```python
from build123d import *

# Parameters (mm, degrees)
SKETCH5_W             = 29.1
SKETCH5_H             = 16.3
SKETCH5_W_2           = 23.1
SKETCH5_H_2           = 10.3
BOSS_EXTRUDE3_DEPTH   = 7.5
FILLET1_R             = 3
SKETCH7_R             = 1
BOSS_EXTRUDE5_DEPTH   = 4
SKETCH11_W            = 10
SKETCH11_H            = 4
BOSS_EXTRUDE6_DEPTH   = 12
FILLET3_R             = 3
SKETCH13_R            = 2.25
CUT_EXTRUDE1_DEPTH    = 34.593154064
CHAMFER2_SIZE         = 1
CHAMFER2_SIZE2        = 1.732050808
CIRPATTERN1_OUTLINE_R = 2.25
CIRPATTERN1_DEPTH     = 2.9999999
CIRPATTERN1_START     = 2.9999999
CIRPATTERN1_2_DEPTH   = 1.0000001
FILLET5_R             = 3
CHAMFER3_SIZE         = 1
CHAMFER3_SIZE2        = 0.577350269


with BuildPart() as part:
    # Sketch5 → Boss-Extrude3 (new body)
    with BuildSketch(Plane(origin=(0, 0, 0), x_dir=(1, 0, 0), z_dir=(0, 1, 0))):
        with Locations((14.55, 8.15)):
            Rectangle(SKETCH5_W, SKETCH5_H)
        with Locations((14.55, 8.15)):
            Rectangle(SKETCH5_W_2, SKETCH5_H_2, mode=Mode.SUBTRACT)
    extrude(amount=BOSS_EXTRUDE3_DEPTH)

    # Fillet1
    fillet1_edges = [part.edges().sort_by_distance(p)[0] for p in [
        (29.1, 3.75, -16.3),
        (29.1, 3.75, 0),
        (0, 3.75, 0),
        (0, 3.75, -16.3),
    ]]
    fillet(fillet1_edges, radius=FILLET1_R)

    # Sketch7 → Boss-Extrude5 (add)
    with BuildSketch(Plane(origin=(0, 0, 0), x_dir=(1, 0, 0), z_dir=(0, 1, 0))):
        with BuildLine():
            Line((5.5, 8.5), (3, 8.5))
            Line((3, 8.5), (3, 2.5))
            Line((3, 2.5), (5.5, 2.5))
            ThreePointArc((5.5, 2.5), (8.5, 5.5), (5.5, 8.5))
        make_face()
        with Locations(Location((5.5, 5.5, 0), (0, 0, 270))):
            Circle(SKETCH7_R, mode=Mode.SUBTRACT)
    extrude(amount=BOSS_EXTRUDE5_DEPTH)

    # Sketch11 → Boss-Extrude6 (add)
    with BuildSketch(Plane.XY):
        with Locations((14.55, 2)):
            Rectangle(SKETCH11_W, SKETCH11_H)
    extrude(amount=BOSS_EXTRUDE6_DEPTH)

    # Fillet3
    fillet3_edges = [part.edges().sort_by_distance(p)[0] for p in [
        (9.55, 2, 0),
        (19.55, 2, 0),
        (14.55, 4, 0),
        (9.55, 2, 12),
        (19.55, 2, 12),
    ]]
    fillet(fillet3_edges, radius=FILLET3_R)

    # Sketch13 → Cut-Extrude1 (cut, through all)
    with BuildSketch(Plane(origin=(0, 4, 0), x_dir=(1, 0, 0), z_dir=(0, 1, 0))):
        with Locations(Location((14.55, -7, 0), (0, 0, 270))):
            Circle(SKETCH13_R)
    extrude(amount=-CUT_EXTRUDE1_DEPTH, mode=Mode.SUBTRACT)

    # Chamfer2
    chamfer2_edges = [part.edges().sort_by_distance(p)[0] for p in [
        (14.55, 4, 4.75),
    ]]
    chamfer2_side = [part.faces().sort_by_distance(p)[0] for p in [
        (14.55, 2, 4.75),
    ]]
    chamfer(chamfer2_edges, length=CHAMFER2_SIZE, length2=CHAMFER2_SIZE2, reference=chamfer2_side[0])

    # CirPattern1: read off the stored shape, not the designer's step
    # CirPattern1 outline → CirPattern1 (add)
    with BuildSketch(Plane(origin=(0, 0, 0), x_dir=(1, 0, 0), z_dir=(0, 1, 0))):
        with BuildLine():
            Line((9.55, 25.3), (9.55, 16.3))
            Line((9.55, 16.3), (19.55, 16.3))
            Line((19.55, 16.3), (19.55, 25.3))
            ThreePointArc((19.55, 25.3), (18.671320344, 27.421320344), (16.55, 28.3))
            Line((16.55, 28.3), (12.55, 28.3))
            ThreePointArc((12.55, 28.3), (10.428679656, 27.421320344), (9.55, 25.3))
        make_face()
        with Locations((14.55, 23.3)):
            Circle(CIRPATTERN1_OUTLINE_R, mode=Mode.SUBTRACT)
    extrude(amount=CIRPATTERN1_DEPTH)

    # CirPattern1 2 outline → CirPattern1 2 (add)
    with BuildSketch(Plane(origin=(0, 0, 0), x_dir=(1, 0, 0), z_dir=(0, 1, 0)).offset(CIRPATTERN1_START)):
        with BuildLine():
            Line((9.55, 25.3), (9.55, 16.3))
            Line((9.55, 16.3), (19.55, 16.3))
            Line((19.55, 16.3), (19.55, 25.3))
            ThreePointArc((19.55, 25.3), (18.671320344, 27.421320344), (16.55, 28.3))
            Line((16.55, 28.3), (12.55, 28.3))
            ThreePointArc((12.55, 28.3), (10.428679656, 27.421320344), (9.55, 25.3))
        make_face()
    extrude(amount=CIRPATTERN1_2_DEPTH)

    # CirPattern1 3 outline → CirPattern1 3 (revolve, cut)
    with BuildSketch(Plane(origin=(14.55, 0, -23.3), x_dir=(1, 0, 0), z_dir=(0, 0, 1))):
        Polygon((0, 2.9999999), (2.25, 2.9999999), (3.982050808, 4), (0, 4), align=None)
    revolve(axis=Axis((14.55, 0, -23.3), (0, 1, 0)), mode=Mode.SUBTRACT)

    # Fillet5
    fillet5_edges = [part.edges().sort_by_distance(p)[0] for p in [
        (19.55, 2, -16.3),
        (9.55, 2, -16.3),
        (14.55, 4, -16.3),
    ]]
    fillet(fillet5_edges, radius=FILLET5_R)

    # Chamfer3
    chamfer3_edges = [part.edges().sort_by_distance(p)[0] for p in [
        (5.5, 4, -6.5),
    ]]
    chamfer3_side = [part.faces().sort_by_distance(p)[0] for p in [
        (8.297810971, 4, -6.343571748),
    ]]
    chamfer(chamfer3_edges, length=CHAMFER3_SIZE, length2=CHAMFER3_SIZE2, reference=chamfer3_side[0])


solid = part.part
```
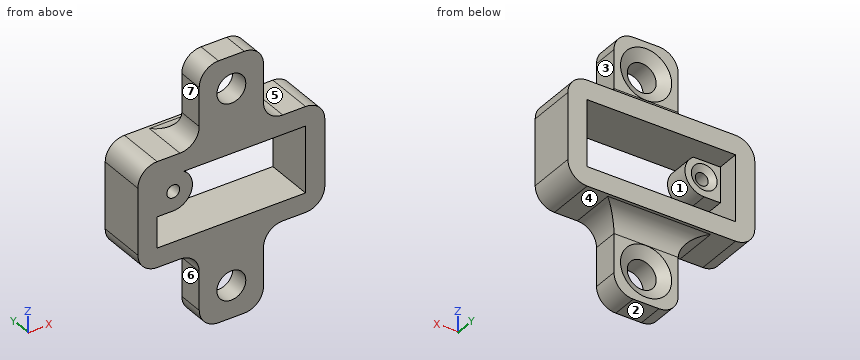
Here's how the part is built. I have some questions about the finished solid (model axes, mm). Face numbers are marked on the shaded views. A direction names the side the tool comes from. Coordinates: 2 decimals unless noted, no trailing zeros. Write each loop counter-clockwise with the first axis right and the second up, starting at its lowest first coordinate (ties: lowest second). Pieces come first, ordered by that corner, then holes. Notation, with made-up numbers: M 84,73 L 129,73 A12 ccw 129,79 Z; hole C 78,34.5 d9. An arc over 180 degrees is marked long. Answer as CSV lines item,"result". Start each with the question number.
Q1. Will these pins go through, and if not, where does the flat tip stop? pin 1 Ø4.5 at (y, z) = (1.5, 6) entering from +X; pin 2 Ø4.5 at (y, z) = (2, 5) entering from -X; pin 3 Ø2 at (x, y) = (11, 3.5) entering from +Z; pin 4 Ø4 at (x, z) = (14.55, 7) entering from -Y.
Q2. Suppose I cut it at C-C, the plane x = 14.55. State how many separate pieces and enclosed holes the cut face has, then the cut area to 3 significant figures.
Q3. I need wall thicknesses on probe 1 along X at (y, z) = (1.6, -5.5); probe 2 along Z at (x, y) = (4.25, 5.75); probe 3 along X at (y, z) = (0.75, -12.5). Which ranges of each line are inside material? Lowest first, please. Write a range as [from, to].
Q4. Suppose I cut it at A-A, the plane x = 24. List the corners of the cut face in (y, z) for me, then the cut area to 3 significant figures.
Q5. Suppose I cut it at B-B, the plane z = -5.5. List the corners of the cut face in (x, y) for me, then the cut area to 3 significant figures.
Q6. Suppose I cut it at D-D, the plane z = -23.3. List the corners of the cut face in (x, y) for me.
Q7. If we mould it in two halves opening along Z, with no side actions, what happens to the marked faces 1, 2 and 3? For each: pulls with the +Z half, pulls with the -Z half, needs draft (parallel to the pull), parting line crosses it, or undercut.
Q8. For the marked faces 4, 5, 6 and 7, which set-ups out of +Z, -Z, +X, -X, +Y, -Y let a thin tool reach every point of the face, with its end or its side?
Entries:
1,pin 1,"stops at x = 19.55"
1,pin 2,"stops at x = 9.54"
1,pin 3,"stops at z = 11.95"
1,pin 4,"passes through"
2,separate pieces,"4"
2,enclosed holes,"0"
2,area,"105 mm²"
3,probe 1,"x = [0, 4.5], [6.5, 8.5], [26.1, 29.1]"
3,probe 2,"z = [-16.3, -13.3], [-3, 0]"
3,probe 3,"x = [0, 3], [26.1, 29.1]"
4,outline,"M 0,-16.3 L 7.5,-16.3 L 7.5,-13.3 L 0,-13.3 Z; M 0,-3 L 7.5,-3 L 7.5,0 L 0,0 Z"
4,area,"45.0 mm²"
5,outline,"M 0,0 L 4.5,0 L 4.5,3.42 L 3.5,4 L 3,4 L 3,7.5 L 0,7.5 Z; M 6.5,0 L 8.5,0 L 8.5,4 L 7.5,4 L 6.5,3.42 Z; M 26.1,0 L 29.1,0 L 29.1,7.5 L 26.1,7.5 Z"
5,area,"58.4 mm²"
6,outline,"M 9.55,0 L 12.3,0 L 12.3,3 L 10.57,4 L 9.55,4 Z; M 16.8,0 L 19.55,0 L 19.55,4 L 18.53,4 L 16.8,3 Z"
7,face 1,"undercut"
7,face 2,"pulls with the -Z half"
7,face 3,"needs draft"
8,face 4,"-Z, +Y"
8,face 5,"+Z, +Y"
8,face 6,"-Z, -X, +Y, -Y"
8,face 7,"+Z, -X, +Y, -Y"
